from build123d import *

# Parameters (mm, degrees)
SKETCH1_R           = 101.6
BOSS_EXTRUDE1_DEPTH = 73.152
SKETCH3_W           = 60.452
SKETCH3_H           = 57.15
SKETCH4_R           = 26.416
CUT_EXTRUDE1_DEPTH  = 73.152


with BuildPart() as part:
    # Sketch1 → Boss-Extrude1 (new body)
    with BuildSketch(Plane.XY):
        Circle(SKETCH1_R)
    extrude(amount=BOSS_EXTRUDE1_DEPTH)

    # Sketch3 → Cut-Revolve2 (revolve, cut)
    with BuildSketch(Plane(origin=(0, 0, 0), x_dir=(0, 0, -1), z_dir=(1, 0, 0))):
        with Locations((-36.576, 73.025)):
            Rectangle(SKETCH3_W, SKETCH3_H)
    revolve(axis=Axis((0, 0, 0), (0, 0, 1)), mode=Mode.SUBTRACT)

    # Sketch4 → Cut-Extrude1 (cut)
    with BuildSketch(Plane(origin=(0, 0, 0), x_dir=(-1, 0, 0), z_dir=(0, 0, -1))):
        Circle(SKETCH4_R)
    extrude(amount=-CUT_EXTRUDE1_DEPTH, mode=Mode.SUBTRACT)


solid = part.part
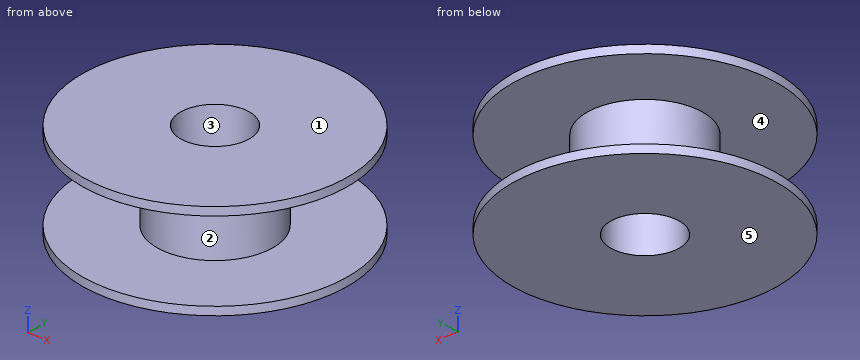
The listing builds one solid part. Answer for the finished solid, in the listing's coordinates (mm). Face numbers are marked on the shaded views. A direction names the side the tool comes from. Round coordinates to 2 decimals unless told otherwise and drop trailing zeros. Write each loop counter-clockwise with the first axis right and the second up, starting at its lowest first coordinate (ties: lowest second). Pieces come first, ordered by that corner, then holes. Notation, with made-up numbers: (-15, 82) - (11, 82) arc R29 ccw to (11, 119) - close; hole circle Ø11 at (50.5, 43). An arc over 180 degrees is marked (long way). Use one line per item in the form item = value. Start each with the question number.
Item 1: A tool of negligible diameter and unlimited length cuts with its end or side. For the marked faces 4 and 5, from which of +Z, -Z, +X, -X, +Y, -Y can it reach the whole face along a straight path? Write none if from no direction.
Item 2: A cutting plane is placed at C-C (z = 43.5). Write down the section's boundary in (x, y).
Item 3: A cutting plane is placed at A-A (y = 0). Write down the section's boundary in (x, z).
Item 4: Flat-ended cylindrical pins translate along their axes: pin 1 Ø6 at (y, z) = (-13.5, 57.5) entering from -X; pin 2 Ø5 at (y, z) = (-7, 17.5) entering from -X. Find the tip coordinate at first contact, or state that the pin passes through.
Item 5: A cutting plane is placed at D-D (x = -49.5). Write down the section's boundary in (y, z).
Item 6: Find the intervals of material crossed by line 1 (Y direction, x = 0, z = 28); line 2 (Z direction, x = -28.5, y = -55); line 3 (X direction, y = 10, z = 11.5), in increasing order. Write a range as [from, to].
Item 7: Determine the mould class of the marked faces 1, 2 and 3 for opening direction X: +X half, -X half, draft (parallel to the pull), parting line (faces both ways), or undercut.
The answers:
q1.face_4 = none
q1.face_5 = -Z, +X, -X, +Y, -Y
q2.outline = circle Ø88.9 at (0, 0); hole circle Ø52.83 at (0, 0)
q3.outline = (-101.6, 0) - (-26.42, 0) - (-26.42, 73.15) - (-101.6, 73.15) - (-101.6, 66.8) - (-44.45, 66.8) - (-44.45, 6.35) - (-101.6, 6.35) - close; (26.42, 0) - (101.6, 0) - (101.6, 6.35) - (44.45, 6.35) - (44.45, 66.8) - (101.6, 66.8) - (101.6, 73.15) - (26.42, 73.15) - close
q4.pin_1 = -43.19
q4.pin_2 = -44.22
q5.outline = (-88.73, 0) - (88.73, 0) - (88.73, 6.35) - (-88.73, 6.35) - close; (-88.73, 66.8) - (88.73, 66.8) - (88.73, 73.15) - (-88.73, 73.15) - close
q6.line_1 = [-44.45, -26.42], [26.42, 44.45]
q6.line_2 = [0, 6.35], [66.8, 73.15]
q6.line_3 = [-43.31, -24.45], [24.45, 43.31]
q7.face_1 = draft
q7.face_2 = parting line
q7.face_3 = undercut
